Source: three-view drawing plus pictorial views. Frame: mm from the lowest corner of the part. Give positions to 0.01 mm unless a question says otherwise; leave off trailing zeros. Order: outer loops, then holes, each group sorted by start corner. A loop starts at its lowest first (then second) coordinate and runs counter-clockwise, first axis right, second up. Notation, with made-up numbers: M 32.5,55 L 55.5,55 A9 cw 55.5,65 Z; hole C -0.75,73 d5. An arc over 180 degrees is marked long. Use CSV: the item, a comma, the result in double quotes. Start each with the question number.
1. Section query D-D, the plane x = 4. Return the cut outline in (y, z).
2. Pin query (flat end, axial travel): P1, Ø1, axis at y = 16.5, z = 0.5, coming from the -X side; P2, Ø1.4, axis at x = 18.5, y = 5.5, coming from the +Z side; P3, Ø1.5, axis at y = 24, z = 3, coming from the +X side; P4, Ø1, axis at x = 29.5, z = 3, coming from the -Y side. Return the tip coordinate at first contact, or that it passes through.
3. Section query A-A, the plane y = 18.5. Return the cut outline in (x, z), plus the area to 3 significant figures.
4. Line query: line 1 along Y through (x, z) = (18.5, 1.75); line 2 along Y through (x, z) = (18, 1.95); line 3 along Y through (x, z) = (7.5, 4.45) (1 decimal). Output: solid intervals per line, ascending. Write a range as [from, to].
5. Section query C-C, the plane z = 2.9. Return the cut outline in (x, y), plus the area to 3 significant figures.
6. Section query B-B, the plane y = 25. Return the cut outline in (x, z).
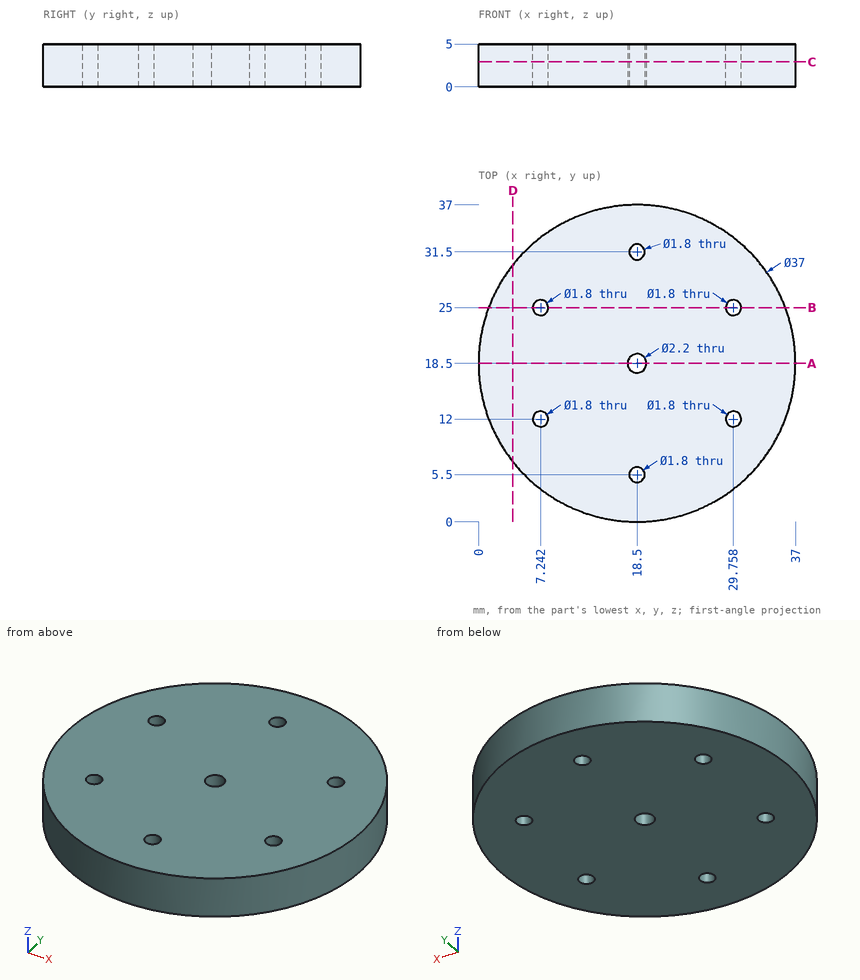
Result set:
1,outline,"M 7.01,0 L 29.99,0 L 29.99,5 L 7.01,5 Z"
2,P1,"x = 0.06"
2,P2,"through"
2,P3,"x = 36.38"
2,P4,"y = 3.27"
3,outline,"M 0,0 L 17.4,0 L 17.4,5 L 0,5 Z; M 19.6,0 L 37,0 L 37,5 L 19.6,5 Z"
3,area,"174 mm2"
4,line 1,"[0, 4.6], [6.4, 17.4], [19.6, 30.6], [32.4, 37]"
4,line 2,"[0.01, 4.75], [6.25, 17.52], [19.48, 30.75], [32.25, 36.99]"
4,line 3,"[3.6, 11.1], [12.9, 24.1], [25.9, 33.4]"
5,outline,"C 18.5,18.5 d37; hole C 7.24,12 d1.8; hole C 7.24,25 d1.8; hole C 18.5,18.5 d2.2; hole C 18.5,5.5 d1.8; hole C 18.5,31.5 d1.8; hole C 29.76,12 d1.8; hole C 29.76,25 d1.8"
5,area,"1,060 mm2"
6,outline,"M 1.18,0 L 6.34,0 L 6.34,5 L 1.18,5 Z; M 8.14,0 L 28.86,0 L 28.86,5 L 8.14,5 Z; M 30.66,0 L 35.82,0 L 35.82,5 L 30.66,5 Z"
